Here's how the part is built. I have some questions about the finished solid (model axes, mm). Round coordinates to 2 decimals unless told otherwise and drop trailing zeros. Write each loop counter-clockwise with the first axis right and the second up, starting at its lowest first coordinate (ties: lowest second). Pieces come first, ordered by that corner, then holes. Notation, with made-up numbers: M -15.5,-23.5 L 9.5,-23.5 A37 cw 9.5,15.5 Z; hole C -15.5,-10 d8. An arc over 180 degrees is marked long. Use one line per item in the form item = value. Start each with the question number.
Q1. We'd pull the mould along Z, two halves only. Please class faces 1 (the face through (56, 0, 6)), 2 (the face through (5.151, 9.392, 7.477)), 3 (the face through (56, 9, 12.7)), 4 (the face through (56, 9, 0)): +Z half, -Z half, draft (parallel to the pull), parting line (faces both ways), or undercut.
Q2. I'm going to push a flat-ended pin straight in: pin 1 Ø1.5 at (y, z) = (3.5, 2) entering from +X. Where does the tip first touch, or does it pass through?
Q3. I want a section at B-B on y = 15.75. List the corners of the cut face in (x, z) for me.
Q4. I need wall thicknesses on line 1 along X through (y, z) = (4.25, 9.25); line 2 along Z through (x, y) = (9, 9.25); line 3 along X through (y, z) = (4.75, 2). Which ranges of each line are inside material? Lowest first, please. Write a range as from..to.
Q5. I want a section at A-A on y = 9. List the corners of the cut face in (x, z) for me, and give its area (3 significant figures).
```python
from build123d import *

# Parameters (mm, degrees)
F0_W     = 114.3
F0_H     = 12.7
F1_DEPTH = 19.05
F3_R     = 5.08
F4_DEPTH = 19.05
F5_R     = 5.08
F7_DEPTH = 25.4
F8_R     = 5.08


with BuildPart() as f1:
    # F0 (on Front) → F1 (new body)
    with BuildSketch(Plane.XZ):
        with Locations((57.15, 6.35)):
            Rectangle(F0_W, F0_H)
    extrude(amount=-F1_DEPTH)

    # F3
    f3_edges = [f1.edges().sort_by_distance(p)[0] for p in [
        (0, 0, 6.35),
    ]]
    fillet(f3_edges, radius=F3_R)

    # F2 (on face) → F4 (cut)
    with BuildSketch(Plane.XZ):
        Polygon((10.16, 6.35), (0, 8.636), (0, 4.064), align=None)
    extrude(amount=-F4_DEPTH, mode=Mode.SUBTRACT)

    # F5
    f5_edges = [f1.edges().sort_by_distance(p)[0] for p in [
        (0, 19.05, 10.668),
        (0, 19.05, 2.032),
    ]]
    fillet(f5_edges, radius=F5_R)

    # F6 (on face) → F7 (cut)
    with BuildSketch(Plane.XZ):
        Polygon((114.3, 3.81), (114.3, 8.89), (106.68, 6.35), align=None)
    extrude(amount=-F7_DEPTH, mode=Mode.SUBTRACT)

    # F8
    f8_edges = [f1.edges().sort_by_distance(p)[0] for p in [
        (114.3, 0, 10.795),
        (114.3, 0, 1.905),
        (114.3, 19.05, 10.795),
        (114.3, 19.05, 1.905),
    ]]
    fillet(f8_edges, radius=F8_R)


solid = f1.part
```
Reported:
q1.face_1 = draft
q1.face_2 = undercut
q1.face_3 = +Z half
q1.face_4 = -Z half
q2.pin_1 = 114.23
q3.outline = M 0.32,0 L 113.98,0 L 113.98,3.92 L 106.68,6.35 L 113.98,8.78 L 113.98,12.7 L 0.32,12.7 L 0.32,8.56 L 10.16,6.35 L 0.32,4.14 Z
q4.line_1 = 0.07..114.23
q4.line_2 = 0..6.09, 6.61..12.7
q4.line_3 = 0.01..114.29
q5.outline = M 0,0 L 114.3,0 L 114.3,3.81 L 106.68,6.35 L 114.3,8.89 L 114.3,12.7 L 0,12.7 L 0,8.64 L 10.16,6.35 L 0,4.06 Z
q5.area = 1,410 mm^2
